Part model, mm, in its own coordinate system. Face numbers are marked on the shaded views. A direction names the side the tool comes from. Coordinates: 2 decimals unless noted, no trailing zeros. Order: outer loops, then holes, each group sorted by start corner. A loop starts at its lowest first (then second) coordinate and runs counter-clockwise, first axis right, second up. Notation, with made-up numbers: M -19,66.25 L 39,66.25 A34 cw 39,104.25 Z; hole C -37,48.5 d2. An arc over 180 degrees is marked long. Write item = value, one per line. Start each with the question number.
from build123d import *

# Parameters (mm, degrees)
SKETCH1_W            = 81.5
SKETCH1_H            = 77
BOSS_EXTRUDE1_DEPTH  = 2
SKETCH2_W            = 81.5
SKETCH2_H            = 6.7
BOSS_EXTRUDE2_DEPTH  = 8
SKETCH3_W            = 22.3
SKETCH3_H            = 6.7
BOSS_EXTRUDE3_DEPTH  = 10
SKETCH4_W            = 53.2
SKETCH4_H            = 6.7
BOSS_EXTRUDE4_DEPTH  = 10
SKETCH5_W            = 81.5
SKETCH5_H            = 1.2
BOSS_EXTRUDE5_DEPTH  = 8
SKETCH6_W            = 22.3
SKETCH6_H            = 1.2
BOSS_EXTRUDE6_DEPTH  = 11
SKETCH7_W            = 53.2
SKETCH7_H            = 1.2
BOSS_EXTRUDE7_DEPTH  = 11
SKETCH8_W            = 81.5
SKETCH8_H            = 6.7
BOSS_EXTRUDE8_DEPTH  = 5
SKETCH9_W            = 59
SKETCH9_H            = 6.7
BOSS_EXTRUDE9_DEPTH  = 10
SKETCH10_W           = 12.5
SKETCH10_H           = 6.7
BOSS_EXTRUDE10_DEPTH = 10
SKETCH11_W           = 81.5
SKETCH11_H           = 1.2
BOSS_EXTRUDE11_DEPTH = 5
SKETCH12_W           = 59
SKETCH12_H           = 1.2
BOSS_EXTRUDE12_DEPTH = 11
SKETCH13_W           = 12.5
SKETCH13_H           = 1.2
BOSS_EXTRUDE13_DEPTH = 11
SKETCH14_W           = 2.2
SKETCH14_H           = 63.6
BOSS_EXTRUDE14_DEPTH = 10
SKETCH15_W           = 1.2
SKETCH15_H           = 61.2
BOSS_EXTRUDE15_DEPTH = 11
SKETCH16_W           = 2.2
SKETCH16_H           = 63.6
BOSS_EXTRUDE16_DEPTH = 5
SKETCH17_W           = 2.2
SKETCH17_H           = 48.3
BOSS_EXTRUDE17_DEPTH = 10
SKETCH18_W           = 2.2
SKETCH18_H           = 7.3
BOSS_EXTRUDE18_DEPTH = 10
SKETCH19_W           = 1.2
SKETCH19_H           = 61.2
BOSS_EXTRUDE19_DEPTH = 5
SKETCH20_W           = 1.2
SKETCH20_H           = 47.1
BOSS_EXTRUDE20_DEPTH = 11
SKETCH21_W           = 1.2
SKETCH21_H           = 6.1
BOSS_EXTRUDE21_DEPTH = 11
SKETCH22_R           = 1.7
CUT_EXTRUDE1_DEPTH   = 17
SKETCH23_R           = 9.3
CUT_EXTRUDE2_DEPTH   = 17
SKETCH24_R           = 1.2
CUT_EXTRUDE3_DEPTH   = 17
SKETCH25_R           = 2
CUT_EXTRUDE4_DEPTH   = 1
SKETCH26_R           = 1.2
CUT_EXTRUDE5_DEPTH   = 17
SKETCH27_R           = 2
CUT_EXTRUDE6_DEPTH   = 1
SKETCH28_R           = 1.2
CUT_EXTRUDE7_DEPTH   = 17
SKETCH29_R           = 2
CUT_EXTRUDE8_DEPTH   = 1
SKETCH30_R           = 1.2
CUT_EXTRUDE9_DEPTH   = 17
SKETCH31_R           = 2
CUT_EXTRUDE10_DEPTH  = 1


with BuildPart() as part:
    # Sketch1 → Boss-Extrude1 (new body)
    with BuildSketch(Plane(origin=(0, 0, 0), x_dir=(0, 1, 0), z_dir=(0, 0, 1))):
        with Locations((40.75, -38.5)):
            Rectangle(SKETCH1_W, SKETCH1_H)
    extrude(amount=BOSS_EXTRUDE1_DEPTH)

    # Sketch2 → Boss-Extrude2 (add)
    with BuildSketch(Plane(origin=(0, 0, 0), x_dir=(0, 1, 0), z_dir=(0, 0, 1))):
        with Locations((40.75, -3.35)):
            Rectangle(SKETCH2_W, SKETCH2_H)
    extrude(amount=BOSS_EXTRUDE2_DEPTH)

    # Sketch3 → Boss-Extrude3 (add)
    with BuildSketch(Plane(origin=(0, 0, 0), x_dir=(0, 1, 0), z_dir=(0, 0, 1))):
        with Locations((11.15, -3.35)):
            Rectangle(SKETCH3_W, SKETCH3_H)
    extrude(amount=BOSS_EXTRUDE3_DEPTH)

    # Sketch4 → Boss-Extrude4 (add)
    with BuildSketch(Plane(origin=(0, 0, 0), x_dir=(0, 1, 0), z_dir=(0, 0, 1))):
        with Locations((54.9, -3.35)):
            Rectangle(SKETCH4_W, SKETCH4_H)
    extrude(amount=BOSS_EXTRUDE4_DEPTH)

    # Sketch5 → Boss-Extrude5 (add)
    with BuildSketch(Plane(origin=(0, 0, 0), x_dir=(0, 1, 0), z_dir=(0, 0, 1))):
        with Locations((40.75, -7.3)):
            Rectangle(SKETCH5_W, SKETCH5_H)
    extrude(amount=BOSS_EXTRUDE5_DEPTH)

    # Sketch6 → Boss-Extrude6 (add)
    with BuildSketch(Plane(origin=(0, 0, 0), x_dir=(0, 1, 0), z_dir=(0, 0, 1))):
        with Locations((11.15, -7.3)):
            Rectangle(SKETCH6_W, SKETCH6_H)
    extrude(amount=BOSS_EXTRUDE6_DEPTH)

    # Sketch7 → Boss-Extrude7 (add)
    with BuildSketch(Plane(origin=(0, 0, 0), x_dir=(0, 1, 0), z_dir=(0, 0, 1))):
        with Locations((54.9, -7.3)):
            Rectangle(SKETCH7_W, SKETCH7_H)
    extrude(amount=BOSS_EXTRUDE7_DEPTH)

    # Sketch8 → Boss-Extrude8 (add)
    with BuildSketch(Plane(origin=(0, 0, 0), x_dir=(0, 1, 0), z_dir=(0, 0, 1))):
        with Locations((40.75, -73.65)):
            Rectangle(SKETCH8_W, SKETCH8_H)
    extrude(amount=BOSS_EXTRUDE8_DEPTH)

    # Sketch9 → Boss-Extrude9 (add)
    with BuildSketch(Plane(origin=(0, 0, 0), x_dir=(0, 1, 0), z_dir=(0, 0, 1))):
        with Locations((29.5, -73.65)):
            Rectangle(SKETCH9_W, SKETCH9_H)
    extrude(amount=BOSS_EXTRUDE9_DEPTH)

    # Sketch10 → Boss-Extrude10 (add)
    with BuildSketch(Plane(origin=(0, 0, 0), x_dir=(0, 1, 0), z_dir=(0, 0, 1))):
        with Locations((75.25, -73.65)):
            Rectangle(SKETCH10_W, SKETCH10_H)
    extrude(amount=BOSS_EXTRUDE10_DEPTH)

    # Sketch11 → Boss-Extrude11 (add)
    with BuildSketch(Plane(origin=(0, 0, 0), x_dir=(0, 1, 0), z_dir=(0, 0, 1))):
        with Locations((40.75, -69.7)):
            Rectangle(SKETCH11_W, SKETCH11_H)
    extrude(amount=BOSS_EXTRUDE11_DEPTH)

    # Sketch12 → Boss-Extrude12 (add)
    with BuildSketch(Plane(origin=(0, 0, 0), x_dir=(0, 1, 0), z_dir=(0, 0, 1))):
        with Locations((29.5, -69.7)):
            Rectangle(SKETCH12_W, SKETCH12_H)
    extrude(amount=BOSS_EXTRUDE12_DEPTH)

    # Sketch13 → Boss-Extrude13 (add)
    with BuildSketch(Plane(origin=(0, 0, 0), x_dir=(0, 1, 0), z_dir=(0, 0, 1))):
        with Locations((75.25, -69.7)):
            Rectangle(SKETCH13_W, SKETCH13_H)
    extrude(amount=BOSS_EXTRUDE13_DEPTH)

    # Sketch14 → Boss-Extrude14 (add)
    with BuildSketch(Plane(origin=(0, 0, 0), x_dir=(0, 1, 0), z_dir=(0, 0, 1))):
        with Locations((1.1, -38.5)):
            Rectangle(SKETCH14_W, SKETCH14_H)
    extrude(amount=BOSS_EXTRUDE14_DEPTH)

    # Sketch15 → Boss-Extrude15 (add)
    with BuildSketch(Plane(origin=(0, 0, 0), x_dir=(0, 1, 0), z_dir=(0, 0, 1))):
        with Locations((2.8, -38.5)):
            Rectangle(SKETCH15_W, SKETCH15_H)
    extrude(amount=BOSS_EXTRUDE15_DEPTH)

    # Sketch16 → Boss-Extrude16 (add)
    with BuildSketch(Plane(origin=(0, 0, 0), x_dir=(0, 1, 0), z_dir=(0, 0, 1))):
        with Locations((80.4, -38.5)):
            Rectangle(SKETCH16_W, SKETCH16_H)
    extrude(amount=BOSS_EXTRUDE16_DEPTH)

    # Sketch17 → Boss-Extrude17 (add)
    with BuildSketch(Plane(origin=(0, 0, 0), x_dir=(0, 1, 0), z_dir=(0, 0, 1))):
        with Locations((80.4, -30.85)):
            Rectangle(SKETCH17_W, SKETCH17_H)
    extrude(amount=BOSS_EXTRUDE17_DEPTH)

    # Sketch18 → Boss-Extrude18 (add)
    with BuildSketch(Plane(origin=(0, 0, 0), x_dir=(0, 1, 0), z_dir=(0, 0, 1))):
        with Locations((80.4, -66.65)):
            Rectangle(SKETCH18_W, SKETCH18_H)
    extrude(amount=BOSS_EXTRUDE18_DEPTH)

    # Sketch19 → Boss-Extrude19 (add)
    with BuildSketch(Plane(origin=(0, 0, 0), x_dir=(0, 1, 0), z_dir=(0, 0, 1))):
        with Locations((78.7, -38.5)):
            Rectangle(SKETCH19_W, SKETCH19_H)
    extrude(amount=BOSS_EXTRUDE19_DEPTH)

    # Sketch20 → Boss-Extrude20 (add)
    with BuildSketch(Plane(origin=(0, 0, 0), x_dir=(0, 1, 0), z_dir=(0, 0, 1))):
        with Locations((78.7, -31.45)):
            Rectangle(SKETCH20_W, SKETCH20_H)
    extrude(amount=BOSS_EXTRUDE20_DEPTH)

    # Sketch21 → Boss-Extrude21 (add)
    with BuildSketch(Plane(origin=(0, 0, 0), x_dir=(0, 1, 0), z_dir=(0, 0, 1))):
        with Locations((78.7, -66.05)):
            Rectangle(SKETCH21_W, SKETCH21_H)
    extrude(amount=BOSS_EXTRUDE21_DEPTH)

    # Sketch22 → Cut-Extrude1 (cut)
    with BuildSketch(Plane(origin=(0, 0, 0), x_dir=(0, 1, 0), z_dir=(0, 0, 1))):
        with Locations(Location((10.7, -29, 0), (0, 0, 270))):
            Circle(SKETCH22_R)
    extrude(amount=CUT_EXTRUDE1_DEPTH, mode=Mode.SUBTRACT)

    # Sketch23 → Cut-Extrude2 (cut)
    with BuildSketch(Plane(origin=(0, 0, 0), x_dir=(0, 1, 0), z_dir=(0, 0, 1))):
        with Locations(Location((64, -38.5, 0), (0, 0, 270))):
            Circle(SKETCH23_R)
    extrude(amount=CUT_EXTRUDE2_DEPTH, mode=Mode.SUBTRACT)

    # Sketch24 → Cut-Extrude3 (cut)
    with BuildSketch(Plane(origin=(0, 0, 0), x_dir=(0, 1, 0), z_dir=(0, 0, 1))):
        with Locations(Location((6, -3.25, 0), (0, 0, 270))):
            Circle(SKETCH24_R)
    extrude(amount=CUT_EXTRUDE3_DEPTH, mode=Mode.SUBTRACT)

    # Sketch25 → Cut-Extrude4 (cut)
    with BuildSketch(Plane(origin=(0, 0, 0), x_dir=(0, 1, 0), z_dir=(0, 0, 1))):
        with Locations(Location((6, -3.25, 0), (0, 0, 270))):
            Circle(SKETCH25_R)
    extrude(amount=CUT_EXTRUDE4_DEPTH, mode=Mode.SUBTRACT)

    # Sketch26 → Cut-Extrude5 (cut)
    with BuildSketch(Plane(origin=(0, 0, 0), x_dir=(0, 1, 0), z_dir=(0, 0, 1))):
        with Locations(Location((75.5, -3.25, 0), (0, 0, 270))):
            Circle(SKETCH26_R)
    extrude(amount=CUT_EXTRUDE5_DEPTH, mode=Mode.SUBTRACT)

    # Sketch27 → Cut-Extrude6 (cut)
    with BuildSketch(Plane(origin=(0, 0, 0), x_dir=(0, 1, 0), z_dir=(0, 0, 1))):
        with Locations(Location((75.5, -3.25, 0), (0, 0, 270))):
            Circle(SKETCH27_R)
    extrude(amount=CUT_EXTRUDE6_DEPTH, mode=Mode.SUBTRACT)

    # Sketch28 → Cut-Extrude7 (cut)
    with BuildSketch(Plane(origin=(0, 0, 0), x_dir=(0, 1, 0), z_dir=(0, 0, 1))):
        with Locations(Location((6, -73.75, 0), (0, 0, 270))):
            Circle(SKETCH28_R)
    extrude(amount=CUT_EXTRUDE7_DEPTH, mode=Mode.SUBTRACT)

    # Sketch29 → Cut-Extrude8 (cut)
    with BuildSketch(Plane(origin=(0, 0, 0), x_dir=(0, 1, 0), z_dir=(0, 0, 1))):
        with Locations(Location((6, -73.75, 0), (0, 0, 270))):
            Circle(SKETCH29_R)
    extrude(amount=CUT_EXTRUDE8_DEPTH, mode=Mode.SUBTRACT)

    # Sketch30 → Cut-Extrude9 (cut)
    with BuildSketch(Plane(origin=(0, 0, 0), x_dir=(0, 1, 0), z_dir=(0, 0, 1))):
        with Locations(Location((75.5, -73.75, 0), (0, 0, 270))):
            Circle(SKETCH30_R)
    extrude(amount=CUT_EXTRUDE9_DEPTH, mode=Mode.SUBTRACT)

    # Sketch31 → Cut-Extrude10 (cut)
    with BuildSketch(Plane(origin=(0, 0, 0), x_dir=(0, 1, 0), z_dir=(0, 0, 1))):
        with Locations(Location((75.5, -73.75, 0), (0, 0, 270))):
            Circle(SKETCH31_R)
    extrude(amount=CUT_EXTRUDE10_DEPTH, mode=Mode.SUBTRACT)


solid = part.part
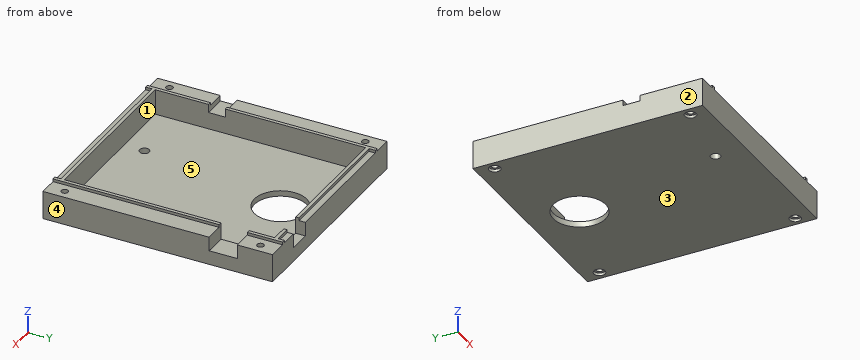
Item 1: Flat gauge pins, fed straight in: pin 1 (1.7 mm diameter, centred on x = 59, y = 79.5, fed in from +Z); pin 2 (0.8 mm diameter, centred on y = 80.5, z = 10.5, fed in from +X); pin 3 (1.2 mm diameter, centred on x = 2.5, y = 5.5, fed in from -Z). Where does each tip first touch, or does it go through?
Item 2: 3-axis set-ups, long thin cutter, end or side, ignore diameter. For the marked faces 1 and 2: which of +Z, -Z, +X, -X, +Y, -Y reach the whole face in a straight line?
Item 3: Pull direction X, two halves, no side cores. Call the marked faces 3, 4 and 5: pulls with the +X half, pulls with the -X half, needs draft (parallel to the pull), parting line crosses it, or undercut.
Item 4: Cut at A-A, the plane y = 10.7. Write the cut outline in (x, z).
Item 5: Wall check: line 1 along Y through (x, z) = (73.75, 4.5); line 2 along Y through (x, z) = (73.75, 8); line 3 along Y through (x, z) = (73.75, 0.4). Give the ranges that are in metal, low to high. Write a range as [from, to].
Item 6: Cut at C-C, the plane y = 75.5. Write the cut outline in (x, z), and give its area (3 significant figures).
Item 7: Cut at D-D, the plane z = 3.5. Write the cut outline in (x, y).
Item 8: Cut at B-B, the plane x = 3.25. Write the cut outline in (y, z), and give its area (3 significant figures).
Filled sheet:
q1.pin_1 = 5
q1.pin_2 = 70.3
q1.pin_3 = 1
q2.face_1 = +Z
q2.face_2 = +Z, -Z, -X, +Y, -Y
q3.face_3 = needs draft
q3.face_4 = pulls with the +X half
q3.face_5 = undercut
q4.outline = M 0,0 L 27.3,0 L 27.3,2 L 7.9,2 L 7.9,11 L 6.7,11 L 6.7,10 L 0,10 Z; M 30.7,0 L 77,0 L 77,10 L 70.3,10 L 70.3,11 L 69.1,11 L 69.1,2 L 30.7,2 Z
q5.line_1 = [0, 4.8], [7.2, 74.3], [76.7, 81.5]
q5.line_2 = [0, 4.8], [7.2, 59], [69, 74.3], [76.7, 81.5]
q5.line_3 = [0, 4], [8, 73.5], [77.5, 81.5]
q6.outline = M 0,0 L 1.25,0 L 1.25,1 L 2.05,1 L 2.05,10 L 0,10 Z; M 4.45,1 L 5.25,1 L 5.25,0 L 71.75,0 L 71.75,1 L 72.55,1 L 72.55,10 L 70.3,10 L 70.3,11 L 69.1,11 L 69.1,2 L 7.9,2 L 7.9,11 L 6.7,11 L 6.7,10 L 4.45,10 Z; M 74.95,1 L 75.75,1 L 75.75,0 L 77,0 L 77,10 L 74.95,10 Z
q6.area = 232 mm2
q7.outline = M 0,0 L 77,0 L 77,81.5 L 0,81.5 Z; hole C 3.25,6 d2.4; hole C 3.25,75.5 d2.4; hole M 7.9,3.4 L 69.1,3.4 L 69.1,78.1 L 7.9,78.1 Z; hole C 73.75,6 d2.4; hole C 73.75,75.5 d2.4
q8.outline = M 0,0 L 4,0 L 4,1 L 4.8,1 L 4.8,10 L 0,10 Z; M 7.2,1 L 8,1 L 8,0 L 73.5,0 L 73.5,1 L 74.3,1 L 74.3,10 L 28.3,10 L 28.3,8 L 22.3,8 L 22.3,10 L 7.2,10 Z; M 76.7,1 L 77.5,1 L 77.5,0 L 81.5,0 L 81.5,10 L 76.7,10 Z
q8.area = 752 mm2
